CAD build for the part. Positions are in the model's coordinates, mm. Face numbers are marked on the shaded views. A direction names the side the tool comes from. Give positions to 0.01 mm unless a question says otherwise; leave off trailing zeros. Write each loop counter-clockwise with the first axis right and the second up, starting at its lowest first coordinate (ties: lowest second). Pieces come first, ordered by that corner, then holes. Notation, with made-up numbers: (7, 42) - (24, 42) arc R32 cw to (24, 72) - close; hole circle Ø4 at (89.5, 42). An arc over 180 degrees is marked (long way). Answer as a JSON object with one key per item and string values.
from build123d import *

# Parameters (mm, degrees)
SKETCH1_W               = 44.4
SKETCH1_H               = 40
SKETCH1_R               = 2.6
BOSS_EXTRUDE1_DEPTH     = 2
SKETCH2_W               = 44.4
SKETCH2_H               = 18.3
BOSS_EXTRUDE2_DEPTH     = 2
LPATTERN1_COUNT         = 2
LPATTERN1_PITCH         = 16.3
SKETCH3_R               = 2.6
CUT_EXTRUDE1_DEPTH      = 64.253853638
CHAMFER1_SIZE           = 1
MIRROR1_COPY_1_SKETCH_W = 44.4
MIRROR1_COPY_1_SKETCH_H = 40
MIRROR1_COPY_1_SKETCH_R = 2.6
MIRROR1_COPY_1_DEPTH    = 2
CHAMFER3_SIZE           = 1


with BuildPart() as part:
    # Sketch1 → Boss-Extrude1 (new body)
    with BuildSketch(Plane.XY):
        with Locations((22.2, 20)):
            Rectangle(SKETCH1_W, SKETCH1_H)
        with Locations((8, 8.476902454)):
            Circle(SKETCH1_R, mode=Mode.SUBTRACT)
        with Locations((8, 29.976902454)):
            Circle(SKETCH1_R, mode=Mode.SUBTRACT)
        with Locations((36.4, 29.976902454)):
            Circle(SKETCH1_R, mode=Mode.SUBTRACT)
        with Locations((36.4, 8.476902454)):
            Circle(SKETCH1_R, mode=Mode.SUBTRACT)
    boss_extrude1 = extrude(amount=BOSS_EXTRUDE1_DEPTH)

    # Sketch2 → Boss-Extrude2 (add)
    with BuildSketch(Plane(origin=(0, 40, 0), x_dir=(1, 0, 0), z_dir=(0, 1, 0))):
        with Locations((22.2, 7.15)):
            Rectangle(SKETCH2_W, SKETCH2_H)
    boss_extrude2 = extrude(amount=BOSS_EXTRUDE2_DEPTH)

    # LPattern1: Boss-Extrude1 ×2
    with Locations(*[(0, 0, -i * LPATTERN1_PITCH) for i in range(1, LPATTERN1_COUNT)]):
        add(boss_extrude1)

    # Sketch3 → Cut-Extrude1 (cut, through all)
    with BuildSketch(Plane(origin=(0, 42, 0), x_dir=(1, 0, 0), z_dir=(0, 1, 0))):
        with Locations(Location((12.2, 7.15, 0), (0, 0, 270))):
            Circle(SKETCH3_R)
        with Locations(Location((32.2, 7.15, 0), (0, 0, 270))):
            Circle(SKETCH3_R)
    extrude(amount=-CUT_EXTRUDE1_DEPTH, mode=Mode.SUBTRACT)

    # Chamfer1
    chamfer1_edges = [part.edges().sort_by_distance(p)[0] for p in [
        (44.4, 21, 2),
        (44.4, 21, -16.3),
        (22.2, 42, 2),
        (44.4, 42, -7.15),
        (22.2, 42, -16.3),
        (22.2, 0, -16.3),
        (0, 0, -15.3),
        (44.4, 0, -15.3),
        (44.4, 0, 1),
        (0, 0, 1),
        (22.2, 0, 2),
    ]]
    chamfer(chamfer1_edges, length=CHAMFER1_SIZE)

    # Mirror1: Boss-Extrude1, Boss-Extrude2 across plane
    add(boss_extrude1.mirror(Plane.ZX.offset(19.226902454)))
    add(boss_extrude2.mirror(Plane.ZX.offset(19.226902454)))

    # Mirror1 copy 1 sketch → Mirror1 copy 1 (add)
    with BuildSketch(Plane(origin=(0, 38.453804908, -16.3), x_dir=(1, 0, 0), z_dir=(0, 0, 1))):
        with Locations((22.2, -20)):
            Rectangle(MIRROR1_COPY_1_SKETCH_W, MIRROR1_COPY_1_SKETCH_H)
        with Locations((8, -8.476902454)):
            Circle(MIRROR1_COPY_1_SKETCH_R, mode=Mode.SUBTRACT)
        with Locations((8, -29.976902454)):
            Circle(MIRROR1_COPY_1_SKETCH_R, mode=Mode.SUBTRACT)
        with Locations((36.4, -29.976902454)):
            Circle(MIRROR1_COPY_1_SKETCH_R, mode=Mode.SUBTRACT)
        with Locations((36.4, -8.476902454)):
            Circle(MIRROR1_COPY_1_SKETCH_R, mode=Mode.SUBTRACT)
    extrude(amount=MIRROR1_COPY_1_DEPTH)

    # Chamfer3
    chamfer3_edges = [part.edges().sort_by_distance(p)[0] for p in [
        (44.4, 17.453804908, 2),
        (44.4, 17.453804908, -16.3),
        (22.2, -3.546195092, -16.3),
        (44.4, -3.546195092, -7.15),
        (22.2, -3.546195092, 2),
    ]]
    chamfer(chamfer3_edges, length=CHAMFER3_SIZE - 0.0001)  # a hair under: the kernel refuses the full size


solid = part.part
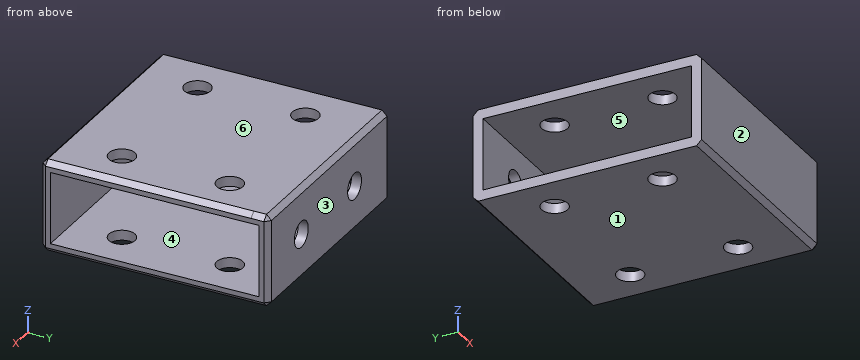
(1) Saw through at D-D, the plane z = -11.5. Give the cut face in (x, y), and give its area (3 significant figures).
Answer key:
{"outline": "(0, -3.55) - (43.4, -3.55) - (44.4, -2.55) - (44.4, -1.55) - (0, -1.55) - close; (0, 40) - (44.4, 40) - (44.4, 41) - (43.4, 42) - (0, 42) - close", "area": "177 mm²"}
(2) Pull direction Y, two halves, no side cores. Call the marked faces 1, 2, 3 and 4: pulls with the +Y half, pulls with the -Y half, needs draft (parallel to the pull), parting line crosses it, or undercut.
Answer key:
{"face 1": "needs draft", "face 2": "pulls with the -Y half", "face 3": "pulls with the +Y half", "face 4": "undercut"}
(3) Probe L1, parallel to Y at x = 8, z = 0.45; L2, parallel to Y at x = 26, z = -9; L3, parallel to Z at x = 26.5, y = 17. List the from-to ranges inside material, lowest first. Write a range as [from, to].
Answer key:
{"L1": "y = [-3.55, 5.88], [11.08, 27.38], [32.58, 42]", "L2": "y = [-3.55, -1.55], [40, 42]", "L3": "z = [-16.3, -14.3], [0, 2]"}
(4) Flat gauge pins, fed straight in: P1, Ø1, axis at x = 37, y = 30, coming from the -Z side; P2, Ø0.8, axis at x = 43.5, z = -16, coming from the +Y side. Where does each tip first touch, or does it go through?
Answer key:
{"P1": "passes through", "P2": "stops at y = 41.69"}
(5) Saw through at C-C, the plane y = 24. Give the cut face in (x, z), and give its area (3 significant figures).
Answer key:
{"outline": "(0, -16.3) - (43.4, -16.3) - (44.4, -15.3) - (44.4, -14.3) - (0, -14.3) - close; (0, 0) - (44.4, 0) - (44.4, 1) - (43.4, 2) - (0, 2) - close", "area": "177 mm²"}
(6) 3-axis set-ups, long thin cutter, end or side, ignore diameter. For the marked faces 5 and 6: which of +Z, -Z, +X, -X, +Y, -Y reach the whole face in a straight line?
Answer key:
{"face 5": "+X, -X", "face 6": "+Z, +X, -X, +Y, -Y"}
(7) Saw through at B-B, the plane x = 8. Give the cut face in (y, z).
Answer key:
{"outline": "(-3.55, -15.3) - (-2.55, -16.3) - (5.88, -16.3) - (5.88, -14.3) - (-1.55, -14.3) - (-1.55, 0) - (5.88, 0) - (5.88, 2) - (-2.55, 2) - (-3.55, 1) - close; (11.08, -16.3) - (27.38, -16.3) - (27.38, -14.3) - (11.08, -14.3) - close; (11.08, 0) - (27.38, 0) - (27.38, 2) - (11.08, 2) - close; (32.58, -16.3) - (41, -16.3) - (42, -15.3) - (42, 1) - (41, 2) - (32.58, 2) - (32.58, 0) - (40, 0) - (40, -14.3) - (32.58, -14.3) - close"}
(8) Saw through at A-A, the plane z = -7.15. Give the cut face in (x, y).
Answer key:
{"outline": "(0, -3.55) - (43.4, -3.55) - (44.4, -2.55) - (44.4, -1.55) - (0, -1.55) - close; (0, 40) - (9.6, 40) - (9.6, 42) - (0, 42) - close; (14.8, 40) - (29.6, 40) - (29.6, 42) - (14.8, 42) - close; (34.8, 40) - (44.4, 40) - (44.4, 41) - (43.4, 42) - (34.8, 42) - close"}
